```python
from build123d import *

# Parameters (mm, degrees)
SKETCH1_R               = 6.35
BOSS_EXTRUDE1_DEPTH     = 51.308
CUT_EXTRUDE1_DEPTH      = 53.087962755
CUT_EXTRUDE1_DEPTH_BACK = 53.087962755
CUT_EXTRUDE2_DEPTH      = 53.087962755
CUT_EXTRUDE2_DEPTH_BACK = 53.087962755


with BuildPart() as part:
    # Sketch1 → Boss-Extrude1 (new body)
    with BuildSketch(Plane(origin=(0, 0, 0), x_dir=(0, 0, -1), z_dir=(1, 0, 0))):
        Circle(SKETCH1_R)
    extrude(amount=BOSS_EXTRUDE1_DEPTH)

    # Sketch2 → Cut-Extrude1 (cut, two sides: drawn at the far end of the back side and taken through both)
    with BuildSketch(Plane(origin=(0, 0, 0), x_dir=(1, 0, 0), z_dir=(0, 1, 0)).offset(-CUT_EXTRUDE1_DEPTH_BACK)):
        Polygon((0, -6.35), (7.332348419, 6.35), (0, 6.35), align=None)
    extrude(amount=CUT_EXTRUDE1_DEPTH + CUT_EXTRUDE1_DEPTH_BACK, mode=Mode.SUBTRACT)

    # Sketch3 → Cut-Extrude2 (cut, two sides: drawn at the far end of the back side and taken through both)
    with BuildSketch(Plane(origin=(0, 0, 0), x_dir=(1, 0, 0), z_dir=(0, 1, 0)).offset(-CUT_EXTRUDE2_DEPTH_BACK)):
        Polygon((33.798828355, -6.35), (41.24323005, 6.35), (51.308, 6.35), (51.308, -6.35), align=None)
    extrude(amount=CUT_EXTRUDE2_DEPTH + CUT_EXTRUDE2_DEPTH_BACK, mode=Mode.SUBTRACT)


solid = part.part
```
CAD build for the part. Positions are in the model's coordinates, mm. Give positions to 0.01 mm unless a question says otherwise; leave off trailing zeros. Write each loop counter-clockwise with the first axis right and the second up, starting at its lowest first coordinate (ties: lowest second). Pieces come first, ordered by that corner, then holes. Notation, with made-up numbers: M 75.5,27 L 121.5,27 A19 ccw 121.5,61 Z; hole C -30.5,-28.5 d4. An arc over 180 degrees is marked long. Return JSON: item names as keys, results as strings. Group by question number.
(1) Band-saw the part on A-A (x = 16). Give the cut face in (y, z), and give its area (3 significant figures).
(2) Band-saw the part on C-C (z = 2.25). Give the cut face in (x, y), and give its area (3 significant figures).
(3) Band-saw the part on B-B (y = 0). Give the cut face in (x, z).
(4) Drill centre lines: L1, parallel to X at y = -5.5, z = 1.25; L2, parallel to X at y = 0.5, z = 1.5; L3, parallel to Y at x = 27, z = -4.25. Where is each one in solid material? Low to high. Write a range as [from, to].
(5) Band-saw the part on D-D (x = 35). Give the cut face in (y, z), and give its area (3 significant figures).
(6) Flat gauge pins, fed straight in: pin 1 Ø4 at (x, y) = (10, 5) entering from +Z; pin 2 Ø2 at (x, y) = (29.5, -3) entering from +Z; pin 3 Ø1.5 at (x, z) = (30, 3) entering from -Y. Where does each tip first touch, or does it go through?
Entries:
{
 "1": {"outline": "C 0,0 d12.7", "area": "127 mm^2"},
 "2": {"outline": "M 2.37,-5.94 L 36.2,-5.94 L 36.2,5.94 L 2.37,5.94 Z", "area": "402 mm^2"},
 "3": {"outline": "M 0,6.35 L 7.33,-6.35 L 41.24,-6.35 L 33.8,6.35 Z"},
 "4": {"L1": "x = [2.94, 36.79]", "L2": "x = [2.8, 36.64]", "L3": "y = [-4.72, 4.72]"},
 "5": {"outline": "M -4.67,4.3 A6.35 ccw long 4.67,4.3 Z", "area": "113 mm^2"},
 "6": {"pin 1": "stops at z = 5.6", "pin 2": "stops at z = 6.03", "pin 3": "stops at y = -5.94"}
}
